Read the model definition and answer for the solid it produces. Units are mm, in the model's axes. A direction names the side the tool comes from. Give positions to 0.01 mm unless a question says otherwise; leave off trailing zeros. Loops run counter-clockwise (first coordinate to the right, second up) from the corner with the lowest first, then second, coordinate; pieces in that order, holes last.
(1) Find section A-A, the plane y = 6.75. Write down the section's boundary in (x, z) (3 decimals).
(2) Find section D-D, the plane z = 3.75. Write down the section's boundary in (x, y).
(3) Which of the six approach directions +Z, -Z, +X, -X, +Y, -Y give full straight-line access (tool end or side, diameter ignored) to faces 5 (the face through (10, 0, 4)), 6 (the face through (-12, 0, 1)), 7 (the face through (-13, -0.1, 0.5))?
(4) Determine the mould class of faces 1 (the face through (12.004, 6.157, 0.507)), 2 (the face through (12.004, -6.157, 0.507)), 3 (the face through (13, -0.1, 0.5)), 4 (the face through (0, -10, 3)) for opening direction Y: pulls with the +Y half, pulls with the -Y half, needs draft (parallel to the pull), parting line crosses it, or undercut.
(5) Straight lines are drawn through the part: probe 1 along Y at (x, z) = (11.23, 0.35) (3 decimals); probe 2 along X at (y, z) = (-6.75, 0.4) (3 decimals); probe 3 along X at (y, z) = (-7.5, 2.25). For each, find the intervals that lie inside material, in ascending order.
(6) Each of these flat-tipped pins is pushed along its axis until it touches: P1, Ø1.5, axis at x = 12, y = -2, coming from the +Z side; P2, Ø1.8, axis at y = 0, z = 4.5, coming from the +X side; P3, Ø1.8, axis at y = 3.5, z = 4.5, coming from the -X side; P4, Ø1.6, axis at x = 11.23, y = 6.75, coming from the +Z side. Where does it stop, or does it pass through?
(7) Find section C-C, the plane y = 2.75. Write down the section's boundary in (x, z), then the cut area to 3 significant figures.
(8) Find section B-B, the plane x = 11.23. Write down the section's boundary in (y, z) (3 decimals).
```python
from build123d import *

# Parameters (mm, degrees)
SKETCH2_W               = 26
SKETCH2_H               = 20
BOSS_EXTRUDE1_DEPTH     = 1
SKETCH3_W               = 20
SKETCH3_H               = 20
BOSS_EXTRUDE2_DEPTH     = 6
SKETCH4_R               = 0.975
CUT_EXTRUDE1_DEPTH      = 2
MIRROR2_COPY_1_SKETCH_R = 0.975
MIRROR2_COPY_1_DEPTH    = 2


with BuildPart() as part:
    # Sketch2 → Boss-Extrude1 (new body)
    with BuildSketch(Plane.XY):
        Rectangle(SKETCH2_W, SKETCH2_H)
    extrude(amount=BOSS_EXTRUDE1_DEPTH)

    # Sketch3 → Boss-Extrude2 (add)
    with BuildSketch(Plane.XY.offset(1)):
        Rectangle(SKETCH3_W, SKETCH3_H)
    extrude(amount=BOSS_EXTRUDE2_DEPTH)

    # Sketch4 → Cut-Extrude1 (cut, through all)
    with BuildSketch(Plane.XY.offset(1)):
        with Locations((-11.23, 6.75)):
            Circle(SKETCH4_R)
    cut_extrude1 = extrude(amount=-CUT_EXTRUDE1_DEPTH, mode=Mode.SUBTRACT)

    # Mirror1: Cut-Extrude1 across plane
    add(cut_extrude1.mirror(Plane(origin=(0, 0, 0), x_dir=(0, 0, 1), z_dir=(1, 0, 0))), mode=Mode.SUBTRACT)

    # Mirror2: Cut-Extrude1 across plane
    add(cut_extrude1.mirror(Plane.ZX), mode=Mode.SUBTRACT)

    # Mirror2 copy 1 sketch → Mirror2 copy 1 (cut, through all)
    with BuildSketch(Plane(origin=(0, 0, 1), x_dir=(-1, 0, 0), z_dir=(0, 0, 1))):
        with Locations((-11.23, 6.75)):
            Circle(MIRROR2_COPY_1_SKETCH_R)
    extrude(amount=-MIRROR2_COPY_1_DEPTH, mode=Mode.SUBTRACT)


solid = part.part
```
Entries:
1. outline: (-13, 0) - (-12.205, 0) - (-12.205, 1) - (-13, 1) - close; (-10.255, 0) - (10.255, 0) - (10.255, 1) - (10, 1) - (10, 7) - (-10, 7) - (-10, 1) - (-10.255, 1) - close; (12.205, 0) - (13, 0) - (13, 1) - (12.205, 1) - close
2. outline: (-10, -10) - (10, -10) - (10, 10) - (-10, 10) - close
3. face 5: +Z, +X, +Y, -Y
3. face 6: +Z, -X, +Y, -Y
3. face 7: +Z, -Z, -X, +Y, -Y
4. face 1: undercut
4. face 2: undercut
4. face 3: needs draft
4. face 4: pulls with the -Y half
5. probe 1: y = -10 to -7.725, -5.775 to 5.775, 7.725 to 10
5. probe 2: x = -13 to -12.205, -10.255 to 10.255, 12.205 to 13
5. probe 3: x = -10 to 10
6. P1: stops at z = 1
6. P2: stops at x = 10
6. P3: stops at x = -10
6. P4: passes through
7. outline: (-13, 0) - (13, 0) - (13, 1) - (10, 1) - (10, 7) - (-10, 7) - (-10, 1) - (-13, 1) - close
7. area: 146 mm2
8. outline: (-10, 0) - (-7.725, 0) - (-7.725, 1) - (-10, 1) - close; (-5.775, 0) - (5.775, 0) - (5.775, 1) - (-5.775, 1) - close; (7.725, 0) - (10, 0) - (10, 1) - (7.725, 1) - close
